Check sheet for the modelled part. Datum: model origin and axes. Units: mm. Face numbers are marked on the shaded views. A direction names the side the tool comes from. Give positions to 0.01 mm unless a question says otherwise; leave off trailing zeros. Order: outer loops, then holes, each group sorted by start corner. A loop starts at its lowest first (then second) coordinate and runs counter-clockwise, first axis right, second up.
Autodesk Inventor part; units mm, degrees
ref_plane "YZ Plane" through (0, 0, 0) normal (1, 0, 0) x (0, 1, 0)
ref_plane "XZ Plane" through (0, 0, 0) normal (0, 1, 0) x (-1, 0, 0)
ref_plane "XY Plane" through (0, 0, 0) normal (0, 0, 1) x (1, 0, 0)
sketch "Sketch1" plane through (0, 0, 0) normal (0, 1, 0) x (-1, 0, 0)
  line L0 (45, 45.3) -> (-45, 45.3)
  line L1 (-45, 45.3) -> (-45, -45.3)
  line L2 (-45, -45.3) -> (45, -45.3)
  line L3 (45, -45.3) -> (45, 45.3)
  line L4 (45, 45.3) -> (-45, -45.3) construction
  line L5 (-45, 45.3) -> (45, -45.3) construction
  point P0 (0, 0)
  dimension "d0" = 90
  dimension "d1" = 90.6
extrude "Extrusion1" add sketch "Sketch1" along normal blind 10
sketch "Sketch2" plane through (-45, 0, 45.3) normal (0, 0, 1) x (1, 0, 0)
  line L0 (90, 10) -> (0, 10)
  line L1 (0, 10) -> (90, 10)
  line L2 (90, 10) -> (90, -80)
  line L3 (90, -80) -> (0, -80)
  line L4 (0, -80) -> (0, 10)
  circle A0 centre (45, -35) radius 45
  circle A1 centre (45, -35) radius 11.5
  point P0 (45, 0)
  point P1 (0, -35)
  point P2 (90, -35)
  dimension "d4" = 90
  dimension "d5" = 90
  dimension "d10" = 23
extrude "Extrusion2" add sketch "Sketch2" along normal blind 10 contours L2 A0 L0 | A0 L4 L0 | A0
extrude "Extrusion4" add sketch "Sketch2" against normal blind 14.5 from surface at -90.6 contours L2 A0 L0 | A0 L4 L0 | A0
sketch "Sketch3" plane through (0, -35, -59.8) normal (0, 0, -1) x (-1, 0, 0)
  circle A0 centre (0, 0) radius 9.4
  circle A1 centre (11.05, 14) radius 2
  circle A2 centre (11.05, -14) radius 2
  circle A3 centre (-28.95, 14) radius 2
  circle A4 centre (-28.95, -14) radius 2
  circle A5 centre (0, 0) radius 8.9
  line L0 (-45, 45) -> (45, 45)
  point P0 (0, 35)
  dimension "d13" = 18.8
  dimension "d14" = 4
  dimension "d15" = 4
  dimension "d16" = 28
  dimension "d17" = 11.05
  dimension "d18" = 14
  dimension "d19" = 4
  dimension "d20" = 4
  dimension "d21" = 40
  dimension "d22" = 40
  dimension "d23" = 14
  dimension "d24" = 28
  dimension "d25" = 14
  dimension "d30" = 0.5
sketch "Sketch4" plane through (0, -35, -45.3) normal (0, 0, 1) x (1, 0, 0)
  circle A0 centre (28.95, 14) radius 2
  circle A1 centre (28.95, -14) radius 2
  circle A2 centre (-11.05, -14) radius 2
  circle A3 centre (-11.05, 14) radius 2
  point P0 (0, 35)
hole "Hole2" at (-11.05, -49, -45.3) at (-11.05, -21, -45.3) at (28.95, -49, -45.3) at (28.95, -21, -45.3) direction (0, 0, -1) diameter 4.134 depth 14.5 counterbore diameter 8 counterbore depth 3
sketch "Sketch5" plane through (0, 0, 0) normal (0, -1, 0) x (1, 0, 0)
  circle A0 centre (-30, -30.3) radius 6.5
  line L0 (-45, -45.3) -> (-45, 45.3)
  line L1 (-45, 0) -> (45, 0)
  line L2 (45, -59.8) -> (45, 55.3)
  line L3 (-45, 45.3) -> (45, 45.3)
  line L4 (0, 45.3) -> (0, -45.3)
  line L5 (45, -45.3) -> (-45, -45.3)
  circle A1 centre (-30, -30.3) radius 2.25
  circle A2 centre (-30, 30.3) radius 6.5
  circle A3 centre (-30, 30.3) radius 2.25
  circle A4 centre (30, -30.3) radius 6.5
  circle A5 centre (30, -30.3) radius 2.25
  circle A6 centre (30, 30.3) radius 2.25
  circle A7 centre (30, 30.3) radius 6.5
  point P0 (0, 0)
  dimension "d59" = 13
  dimension "d60" = 15
  dimension "d61" = 15
  dimension "d62" = 4.5
extrude "Extrusion6" cut sketch "Sketch5" against normal blind 2 contours A0 | A2 | A4 | A7
extrude "Extrusion7" cut sketch "Sketch5" against normal through all contours A1 | A3 | A5 | A6
sketch "Sketch6" plane through (45, -35, 55.3) normal (1, 0, 0) x (0, 0, -1)
  line L0 (7.6158, 13.5) -> (-7.6158, 13.5)
  line L1 (115.1, 0) -> (128.6, 0)
  line L2 (115.1, 0) -> (100.6, 0)
  line L3 (115.1, -11.5) -> (115.1, 11.5)
  circle A0 centre (128.6, 0) radius 15.5
  line L4 (115.1, 45) -> (115.1, 0)
  line L5 (115.1, 7.6158) -> (115.1, -7.6158)
  point P0 (55.3, 35)
extrude "Extrusion8" cut sketch "Sketch6" against normal blind 20
properties part number "Holder2.2"
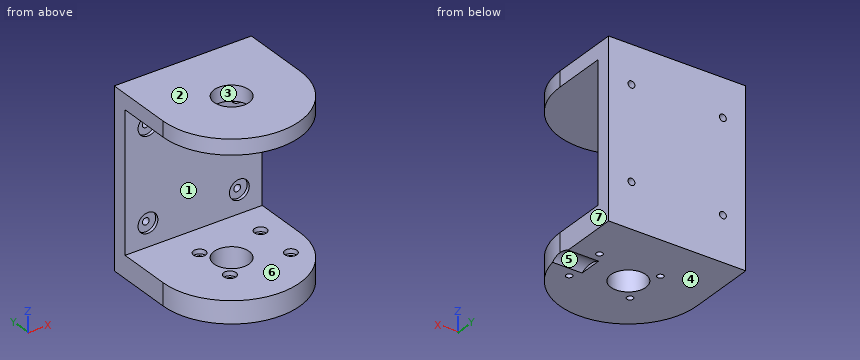
(1) Gauge pin test, flat ends, axial feed: pin 1 Ø4 at (x, z) = (32.5, 27.5) entering from -Y; pin 2 Ø4 at (x, z) = (-30, -30.3) entering from +Y; pin 3 Ø10 at (x, z) = (-8.5, -33.5) entering from -Y; pin 4 Ø2.5 at (x, y) = (28.95, -49) entering from -Z. Record the tip position at first contact, or that the pin passes through.
Response values:
pin 1: stops at y = 2
pin 2: passes through
pin 3: stops at y = 0
pin 4: stops at z = 45.3
(2) Cross-section at C-C on x = 8. Enter the section's corners in (y, z).
Response values:
outline: (-79.28, -59.8) - (-43.26, -59.8) - (-43.26, -45.3) - (-79.28, -45.3) - close; (-79.28, 45.3) - (-43.26, 45.3) - (-43.26, 55.3) - (-79.28, 55.3) - close; (-26.74, -59.8) - (10, -59.8) - (10, 55.3) - (-26.74, 55.3) - (-26.74, 45.3) - (0, 45.3) - (0, -45.3) - (-26.74, -45.3) - close
(3) Material ranges on L1, parallel to Z at x = 30, y = 0.6; L2, parallel to Z at x = 21.5, y = -16.5; L3, parallel to X at y = -21, z = -46, recorded low to high.
Response values:
L1: z = -59.8 to -36.8, -23.8 to 23.8, 36.8 to 55.3
L2: z = -59.8 to -45.3, 45.3 to 55.3
L3: x = -45 to -15.05, -7.05 to 24.95, 32.95 to 45
(4) Cross-section at B-B on y = -21. Enter the section's corners in (x, z).
Response values:
outline: (-45, -59.8) - (-13.12, -59.8) - (-13.12, -48.3) - (-15.05, -48.3) - (-15.05, -45.3) - (-45, -45.3) - close; (-45, 45.3) - (45, 45.3) - (45, 55.3) - (-45, 55.3) - close; (-8.98, -59.8) - (26.88, -59.8) - (26.88, -48.3) - (24.95, -48.3) - (24.95, -45.3) - (-7.05, -45.3) - (-7.05, -48.3) - (-8.98, -48.3) - close; (31.02, -59.8) - (45, -59.8) - (45, -45.3) - (32.95, -45.3) - (32.95, -48.3) - (31.02, -48.3) - close
(5) Set-up check for the marked faces 5, 6 and 7: record each of +Z, -Z, +X, -X, +Y, -Y from which the full face is reachable in a straight line by a thin tool's end or side.
Response values:
face 5: -Z, +X
face 6: +X, -X, -Y
face 7: +Z, -Z, +X, +Y, -Y
(6) Cross-section at D-D on y = -59. Enter the section's corners in (x, z), then the cut area to 3 significant figures.
Response values:
outline: (-38.07, -59.8) - (38.07, -59.8) - (38.07, -45.3) - (-38.07, -45.3) - close; (-38.07, 45.3) - (38.07, 45.3) - (38.07, 55.3) - (-38.07, 55.3) - close
area: 1,870 mm2
(7) Cross-section at A-A on z = 30.3. Enter the section's corners in (x, y), then the cut area to 3 significant figures.
Response values:
outline: (-45, 0) - (-36.5, 0) - (-36.5, 2) - (-32.25, 2) - (-32.25, 10) - (-45, 10) - close; (-27.75, 2) - (-23.5, 2) - (-23.5, 0) - (23.5, 0) - (23.5, 2) - (27.75, 2) - (27.75, 10) - (-27.75, 10) - close; (32.25, 2) - (36.5, 2) - (36.5, 0) - (45, 0) - (45, 10) - (32.25, 10) - close
area: 776 mm2
(8) Release check for a two-part mould opening along Z. For the marked faces 1, 2, 3 and 4 record: released by +Z, released by -Z, zero draft, split by the parting line, or undercut.
Response values:
face 1: undercut
face 2: released by +Z
face 3: zero draft
face 4: released by -Z
